```python
from build123d import *

# Parameters (mm, degrees)
EXTRU_MINCE1_DEPTH                          = 46.5
ESQUISSE2_W                                 = 43
ESQUISSE2_H                                 = 3
BOSS_EXTRU_1_DEPTH                          = 43
ENL_V_MAT_EXTRU_1_REACH                     = 48.5
ESQUISSE3_R                                 = 1.5
FRAISAGE_POUR_VIS_T_TE_FRAIS_E_M41_AT_COUNT = 2
FRAISAGE_POUR_VIS_T_TE_FRAIS_E_M41_AT_PITCH = 71.121375127
FRAISAGE_POUR_VIS_T_TE_FRAIS_E_M41_2_COUNT  = 2
FRAISAGE_POUR_VIS_T_TE_FRAIS_E_M41_2_PITCH  = 66
FRAISAGE_POUR_VIS_T_TE_FRAIS_E_M41_3_COUNT  = 2
FRAISAGE_POUR_VIS_T_TE_FRAIS_E_M41_3_PITCH  = 26.5
ESQUISSE6_W                                 = 25
ESQUISSE6_H                                 = 15
ENL_V_MAT_EXTRU_2_DEPTH                     = 5


with BuildPart() as part:
    # Esquisse1 → Extru.-Mince1 (new body)
    with BuildSketch(Plane.XY):
        Polygon((20, 43), (0, 43), (0, 0), (-43, 0), (-43, 43), (-63, 43), (-63, 40), (-46, 40), (-46, -3), (3, -3), (3, 40), (20, 40), align=None)
    extrude(amount=EXTRU_MINCE1_DEPTH)

    # Esquisse2 → Boss.-Extru.1 (add)
    with BuildSketch(Plane(origin=(0, 0, 0), x_dir=(1, 0, 0), z_dir=(0, 1, 0))):
        with Locations((-21.5, -1.5)):
            Rectangle(ESQUISSE2_W, ESQUISSE2_H)
        with Locations((-21.5, -45)):
            Rectangle(ESQUISSE2_W, ESQUISSE2_H)
    extrude(amount=BOSS_EXTRU_1_DEPTH)

    # Esquisse3 → Enlèv. mat.-Extru.1 (cut, up to next)
    with BuildSketch(Plane.XY.offset(46.5), mode=Mode.PRIVATE) as enl_v_mat_extru_1_sk1:
        with Locations((-37, 4.5)):
            Circle(ESQUISSE3_R)
    enl_v_mat_extru_1_tool1 = extrude(enl_v_mat_extru_1_sk1.sketch, amount=-ENL_V_MAT_EXTRU_1_REACH, mode=Mode.PRIVATE) & part.part
    add(enl_v_mat_extru_1_tool1.solids().sort_by_distance((-37, 4.5, 46.5))[0], mode=Mode.SUBTRACT)
    # Esquisse3 → Enlèv. mat.-Extru.1 (cut, up to next)
    with BuildSketch(Plane.XY.offset(46.5), mode=Mode.PRIVATE) as enl_v_mat_extru_1_sk2:
        with Locations((-37, 35.5)):
            Circle(ESQUISSE3_R)
    enl_v_mat_extru_1_tool2 = extrude(enl_v_mat_extru_1_sk2.sketch, amount=-ENL_V_MAT_EXTRU_1_REACH, mode=Mode.PRIVATE) & part.part
    add(enl_v_mat_extru_1_tool2.solids().sort_by_distance((-37, 35.5, 46.5))[0], mode=Mode.SUBTRACT)
    # Esquisse3 → Enlèv. mat.-Extru.1 (cut, up to next)
    with BuildSketch(Plane.XY.offset(46.5), mode=Mode.PRIVATE) as enl_v_mat_extru_1_sk3:
        with Locations((-6, 35.5)):
            Circle(ESQUISSE3_R)
    enl_v_mat_extru_1_tool3 = extrude(enl_v_mat_extru_1_sk3.sketch, amount=-ENL_V_MAT_EXTRU_1_REACH, mode=Mode.PRIVATE) & part.part
    add(enl_v_mat_extru_1_tool3.solids().sort_by_distance((-6, 35.5, 46.5))[0], mode=Mode.SUBTRACT)
    # Esquisse3 → Enlèv. mat.-Extru.1 (cut, up to next)
    with BuildSketch(Plane.XY.offset(46.5), mode=Mode.PRIVATE) as enl_v_mat_extru_1_sk4:
        with Locations((-6, 4.5)):
            Circle(ESQUISSE3_R)
    enl_v_mat_extru_1_tool4 = extrude(enl_v_mat_extru_1_sk4.sketch, amount=-ENL_V_MAT_EXTRU_1_REACH, mode=Mode.PRIVATE) & part.part
    add(enl_v_mat_extru_1_tool4.solids().sort_by_distance((-6, 4.5, 46.5))[0], mode=Mode.SUBTRACT)
    # Esquisse3 → Enlèv. mat.-Extru.1 (cut, up to next)
    with BuildSketch(Plane.XY.offset(46.5), mode=Mode.PRIVATE) as enl_v_mat_extru_1_sk5:
        with BuildLine():
            Line((-34, 43), (-9, 43))
            Line((-9, 43), (-9, 22))
            ThreePointArc((-9, 22), (-21.5, 9.5), (-34, 22))
            Line((-34, 22), (-34, 43))
        make_face()
    enl_v_mat_extru_1_tool5 = extrude(enl_v_mat_extru_1_sk5.sketch, amount=-ENL_V_MAT_EXTRU_1_REACH, mode=Mode.PRIVATE) & part.part
    add(enl_v_mat_extru_1_tool5.solids().sort_by_distance((-21.5, 27.464973, 46.5))[0], mode=Mode.SUBTRACT)

    # Esquisse5 → Fraisage pour vis à tête fraisée M41 (revolve, cut)
    with BuildSketch(Plane(origin=(-54.5, 40, 36.5), x_dir=(0, 0, -1), z_dir=(1, 0, 0))):
        Polygon((0, 0), (0, 3), (2.275, 3), (2.15, 2.875), (2.15, 2.55), (4.7, 0), align=None)
    fraisage_pour_vis_t_te_frais_e_m41 = revolve(axis=Axis((-54.5, 33.65, 36.5), (0, 1, 0)), mode=Mode.SUBTRACT)

    # Fraisage pour vis à tête fraisée M41 at: Fraisage pour vis à tête fraisée M41 ×2
    with Locations(*[Vector(0.927991056, 0, -0.372602469) * (i * FRAISAGE_POUR_VIS_T_TE_FRAIS_E_M41_AT_PITCH) for i in range(1, FRAISAGE_POUR_VIS_T_TE_FRAIS_E_M41_AT_COUNT)]):
        add(fraisage_pour_vis_t_te_frais_e_m41, mode=Mode.SUBTRACT)

    # Fraisage pour vis _ t_te frais_e M41 2: Fraisage pour vis à tête fraisée M41 ×2
    with Locations(*[(i * FRAISAGE_POUR_VIS_T_TE_FRAIS_E_M41_2_PITCH, 0, 0) for i in range(1, FRAISAGE_POUR_VIS_T_TE_FRAIS_E_M41_2_COUNT)]):
        add(fraisage_pour_vis_t_te_frais_e_m41, mode=Mode.SUBTRACT)

    # Fraisage pour vis _ t_te frais_e M41 3: Fraisage pour vis à tête fraisée M41 ×2
    with Locations(*[(0, 0, -i * FRAISAGE_POUR_VIS_T_TE_FRAIS_E_M41_3_PITCH) for i in range(1, FRAISAGE_POUR_VIS_T_TE_FRAIS_E_M41_3_COUNT)]):
        add(fraisage_pour_vis_t_te_frais_e_m41, mode=Mode.SUBTRACT)

    # Esquisse6 → Enlèv. mat.-Extru.2 (cut)
    with BuildSketch(Plane.XZ.offset(3)):
        with Locations((-21.5, 7.5)):
            Rectangle(ESQUISSE6_W, ESQUISSE6_H)
    extrude(amount=-ENL_V_MAT_EXTRU_2_DEPTH, mode=Mode.SUBTRACT)


solid = part.part
```
Source: CAD feature listing. Evaluate the final solid. Frame: model axes, mm. A direction names the side the tool comes from. Round coordinates to 2 decimals unless told otherwise and drop trailing zeros. Loops run counter-clockwise (first coordinate to the right, second up) from the corner with the lowest first, then second, coordinate; pieces in that order, holes last.
(1) Access query for faces 1 (the flat face through (-22, 7, 43.5)), 2 (the flat face through (-9, 33, 45)), 3 (the flat face through (-46, 19, 23)). Directions: +Z, -Z, +X, -X, +Y, -Y. A direction counts if a zero-diameter tool reaches every point of the face in a straight line with its end or side. Return the directions, or none.
From the geometry:
face 1: +Y
face 2: +Z, +Y
face 3: +Z, -Z, -X, -Y
(2) Pull-direction query (Z, two-part tool) for faces 4 (the flat face through (-22, 25, 0)), 5 (the flat face through (11, 40, 23)), 6 (the cylindrical face through (-56.31, 42.71, 8.84)); classes: +Z half, -Z half, draft (parallel to the pull), parting line (faces both ways), or undercut.
From the geometry:
face 4: -Z half
face 5: draft
face 6: undercut
(3) Contact query for flat-ended pins moving along their axis: pin 1 Ø6 at (y, z) = (34.5, 33) entering from +X; pin 2 Ø10 at (x, y) = (10.5, 38) entering from -Z; pin 3 Ø8.5 at (x, z) = (-58.5, 27) entering from -Y; pin 4 Ø2.5 at (y, z) = (0.5, 10.5) entering from -X. Output: stop coordinate, or through.
From the geometry:
pin 1: stops at x = 3
pin 2: stops at z = 0
pin 3: stops at y = 40
pin 4: stops at x = -46
(4) Section query B-B (x = -21.5). Output: boundary loops of the cut face in (y, z), and give its area (3 significant figures).
From the geometry:
outline: (-3, 15) - (0, 15) - (0, 43.5) - (9.5, 43.5) - (9.5, 46.5) - (-3, 46.5) - close; (2, 0) - (43, 0) - (43, 3) - (2, 3) - close
area: 246 mm2
(5) Material intervals for probe 1 along Y at (x, z) = (-6, 45.45); probe 2 along X at (y, z) = (42.8, 36.5); probe 3 along X at (y, z) = (11.5, 23), sorted ascending.
From the geometry:
probe 1: y = -3 to 3, 6 to 34, 37 to 43
probe 2: x = -63 to -56.65, -52.35 to -43, 0 to 9.35, 13.65 to 20
probe 3: x = -46 to -43, 0 to 3
(6) Section query C-C (y = 4.5). Output: boundary loops of the cut face in (x, z), and give its area (3 significant figures).
From the geometry:
outline: (-46, 0) - (3, 0) - (3, 46.5) - (-4.5, 46.5) - (-4.5, 43.5) - (0, 43.5) - (0, 3) - (-43, 3) - (-43, 43.5) - (-38.5, 43.5) - (-38.5, 46.5) - (-46, 46.5) - close; (-35.5, 43.5) - (-7.5, 43.5) - (-7.5, 46.5) - (-35.5, 46.5) - close
area: 519 mm2
(7) Section query D-D (x = -37). Output: boundary loops of the cut face in (y, z).
From the geometry:
outline: (-3, 0) - (43, 0) - (43, 3) - (0, 3) - (0, 43.5) - (3, 43.5) - (3, 46.5) - (-3, 46.5) - close; (6, 43.5) - (34, 43.5) - (34, 46.5) - (6, 46.5) - close; (37, 43.5) - (43, 43.5) - (43, 46.5) - (37, 46.5) - close
(8) Section query A-A (y = 35.5). Output: boundary loops of the cut face in (x, z), and give its area (3 significant figures).
From the geometry:
outline: (-46, 0) - (3, 0) - (3, 46.5) - (-4.5, 46.5) - (-4.5, 43.5) - (0, 43.5) - (0, 3) - (-43, 3) - (-43, 43.5) - (-38.5, 43.5) - (-38.5, 46.5) - (-46, 46.5) - close; (-35.5, 43.5) - (-34, 43.5) - (-34, 46.5) - (-35.5, 46.5) - close; (-9, 43.5) - (-7.5, 43.5) - (-7.5, 46.5) - (-9, 46.5) - close
area: 444 mm2
